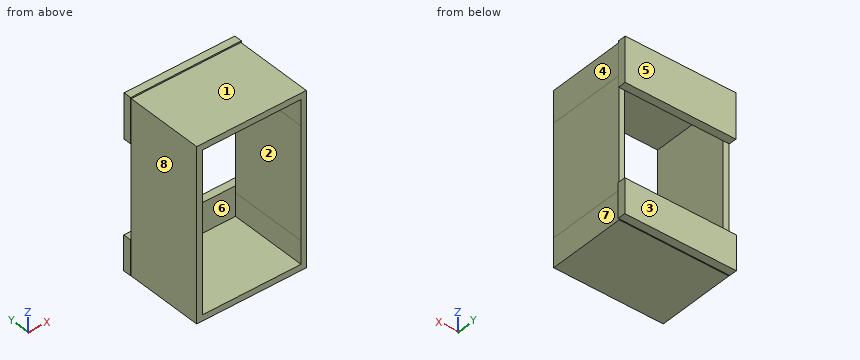
from build123d import *

# Parameters (mm, degrees)
F0_W     = 3.624996
F0_H     = 71.177084
F0_W_2   = 3.375001
F1_DEPTH = 50
F2_DEPTH = 25
F3_W     = 70.750002
F3_H     = 28.750004
F3_W_2   = 71.250003
F3_H_2   = 22.250004
F4_DEPTH = 5


with BuildPart() as f1:
    # F0 (on Front) → F1 (new body)
    with BuildSketch(Plane.XZ):
        Polygon((34.25, 55.528098), (-35.75, 55.528098), (-35.75, 35.21125), (-32.125004, 35.21125), (-32.125004, 51.622394), (30.874999, 51.622394), (30.874999, 35.21125), (34.25, 35.21125), align=None)
        with Locations((-33.937502, -0.377292)):
            Rectangle(F0_W, F0_H)
        with Locations((32.5625, -0.377292)):
            Rectangle(F0_W_2, F0_H)
        Polygon((-32.125004, -35.965834), (-35.75, -35.965834), (-35.75, -54.471902), (34.25, -54.471902), (34.25, -35.965834), (30.874999, -35.965834), (30.874999, -50.627608), (-32.125004, -50.627608), align=None)
    extrude(amount=F1_DEPTH)

    # F0 (on Front) → F2 (join)
    with BuildSketch(Plane.XZ):
        Polygon((34.25, 55.528098), (-35.75, 55.528098), (-35.75, 35.21125), (-32.125004, 35.21125), (-32.125004, 51.622394), (30.874999, 51.622394), (30.874999, 35.21125), (34.25, 35.21125), align=None)
        with Locations((-33.937502, -0.377292)):
            Rectangle(F0_W, F0_H)
        with Locations((32.5625, -0.377292)):
            Rectangle(F0_W_2, F0_H)
        Polygon((-32.125004, -35.965834), (-35.75, -35.965834), (-35.75, -54.471902), (34.25, -54.471902), (34.25, -35.965834), (30.874999, -35.965834), (30.874999, -50.627608), (-32.125004, -50.627608), align=None)
    extrude(amount=F2_DEPTH)

    # F3 (on Front) → F4 (join)
    with BuildSketch(Plane.XZ):
        with Locations((-0.75, 41.997398)):
            Rectangle(F3_W, F3_H)
        with Locations((-0.75, -42.752605)):
            Rectangle(F3_W_2, F3_H_2)
    extrude(amount=-F4_DEPTH)


solid = f1.part
Read the model definition and answer for the solid it produces. Units are mm, in the model's axes. Face numbers are marked on the shaded views. A direction names the side the tool comes from. Coordinates: 2 decimals unless noted, no trailing zeros. Order: outer loops, then holes, each group sorted by start corner. A loop starts at its lowest first (then second) coordinate and runs counter-clockwise, first axis right, second up. Notation, with made-up numbers: (-38.5, 75.25) - (12.5, 75.25) arc R13 cw to (12.5, 99.25) - close; hole circle Ø2 at (-15.75, -24.5). An arc over 180 degrees is marked (long way). Use one line per item in the form item = value.
(1) Which of the six approach directions +Z, -Z, +X, -X, +Y, -Y give full straight-line access (tool end or side, diameter ignored) to the marked faces 1, 2, 3 and 4?
Computed values:
face_1 = +Z, +X, -X, -Y
face_2 = -Y
face_3 = +Z, -Z, +X, -X, +Y
face_4 = +Z, -Z, +X, -Y
(2) Section D-D, the plane z = 33.5 is taken. Give the vertices of the cut face in (x, y) (3 decimals).
Computed values:
outline = (-36.125, 0) - (-35.75, 0) - (-35.75, -50) - (-32.125, -50) - (-32.125, 0) - (30.875, 0) - (30.875, -50) - (34.25, -50) - (34.25, 0) - (34.625, 0) - (34.625, 5) - (-36.125, 5) - close
(3) Straight lines are drawn through the part: L1, parallel to Z at x = -21.5, y = -20; L2, parallel to X at y = -42.5, z = 23.5 (3 decimals). For each, find the intervals that lie inside material, in ascending order.
Computed values:
L1 = -54.47 to -50.63, 51.62 to 55.53
L2 = -35.75 to -32.125, 30.875 to 34.25
(4) Section B-B, the plane x = 12 is taken. Give the vertices of the cut face in (y, z), then the cut area to 4 significant figures.
Computed values:
outline = (-50, -54.47) - (0, -54.47) - (0, -53.88) - (5, -53.88) - (5, -31.63) - (0, -31.63) - (0, -50.63) - (-50, -50.63) - close; (-50, 51.62) - (0, 51.62) - (0, 27.62) - (5, 27.62) - (5, 56.37) - (0, 56.37) - (0, 55.53) - (-50, 55.53) - close
area = 642.5 mm²
(5) For a pull along X with two mould halves and no side action, classify the marked faces 5, 6, 7 and 8 as pulls with the +X half, pulls with the -X half, needs draft (parallel to the pull), parting line crosses it, or undercut.
Computed values:
face_5 = needs draft
face_6 = undercut
face_7 = pulls with the +X half
face_8 = pulls with the -X half
(6) Section A-A, the plane z = -9 is taken. Give the vertices of the cut face in (x, y) (3 decimals), then the cut area to 3 significant figures.
Computed values:
outline = (-35.75, -50) - (-32.125, -50) - (-32.125, 0) - (-35.75, 0) - close; (30.875, -50) - (34.25, -50) - (34.25, 0) - (30.875, 0) - close
area = 350 mm²
(7) Section C-C, the plane y = -39.5 is taken. Give the vertices of the cut face in (x, z) (3 decimals), then the cut area to 3 significant figures.
Computed values:
outline = (-35.75, -54.472) - (34.25, -54.472) - (34.25, 55.528) - (-35.75, 55.528) - close; hole (-32.125, -50.628) - (30.875, -50.628) - (30.875, 51.622) - (-32.125, 51.622) - close
area = 1,260 mm²
(8) Given pin 1 Ø14.5 at (x, z) = (-12.5, 40.5) entering from -Y; pin 2 Ø25 at (y, z) = (-29.5, 3.5) entering from +X; pin 3 Ø1.1 at (x, z) = (-33.5, 2) entering from +Y; pin 4 Ø12 at (x, z) = (-18, -23) entering from -Y, each flat-ended and moving along its own axis, determine where each tip first touches the part or whether it passes through.
Computed values:
pin_1 = 0
pin_2 = 34.25
pin_3 = 0
pin_4 = through
